Check sheet for the drawn part. Datum: minimum x, y, z corner. Units: mm. A direction names the side the tool comes from. Round coordinates to 2 decimals unless told otherwise and drop trailing zeros. Write each loop counter-clockwise with the first axis right and the second up, starting at its lowest first coordinate (ties: lowest second). Pieces come first, ordered by that corner, then holes. Notation, with made-up numbers: (15.5, 11) - (29.5, 11) arc R16 ccw to (29.5, 39) - close; hole circle Ø3 at (-32.5, 59.25). An arc over 180 degrees is marked (long way). Answer as a JSON object with one key per item and string values. Group by question number.
1) Section check C-C (z = 1.1). Enter the section's corners in (x, y), then the cut area to 3 significant figures.
2) Section check D-D (y = 1.2). Enter the section's corners in (x, z), then the cut area to 3 significant figures.
3) Go/stop test with flat-tipped pins: pin 1 Ø1.5 at (y, z) = (2, 2) entering from +X; pin 2 Ø1 at (x, y) = (4.5, 2) entering from -Z. Record where each tip stops, or that it passes through.
4) Thickness scan on line 1 (Y direction, x = 3, z = 1.8); line 2 (Z direction, x = 3.85, y = 5.5); line 3 (Y direction, x = 1.8, z = 1.6). Record the ranges inside material, lowest first.
5) Set-up check for the marked faces 3 and 4: record each of +Z, -Z, +X, -X, +Y, -Y from which the full face is reachable in a straight line by a thin tool's end or side.
6) Mould release check, pull along Y, two halves, no side actions. Record for the marked faces 1 and 2: +Y half, -Y half, draft (parallel to the pull), parting line (faces both ways), or undercut.
7) Section check A-A (y = 3). Enter the section's corners in (x, z), then the cut area to 3 significant figures.
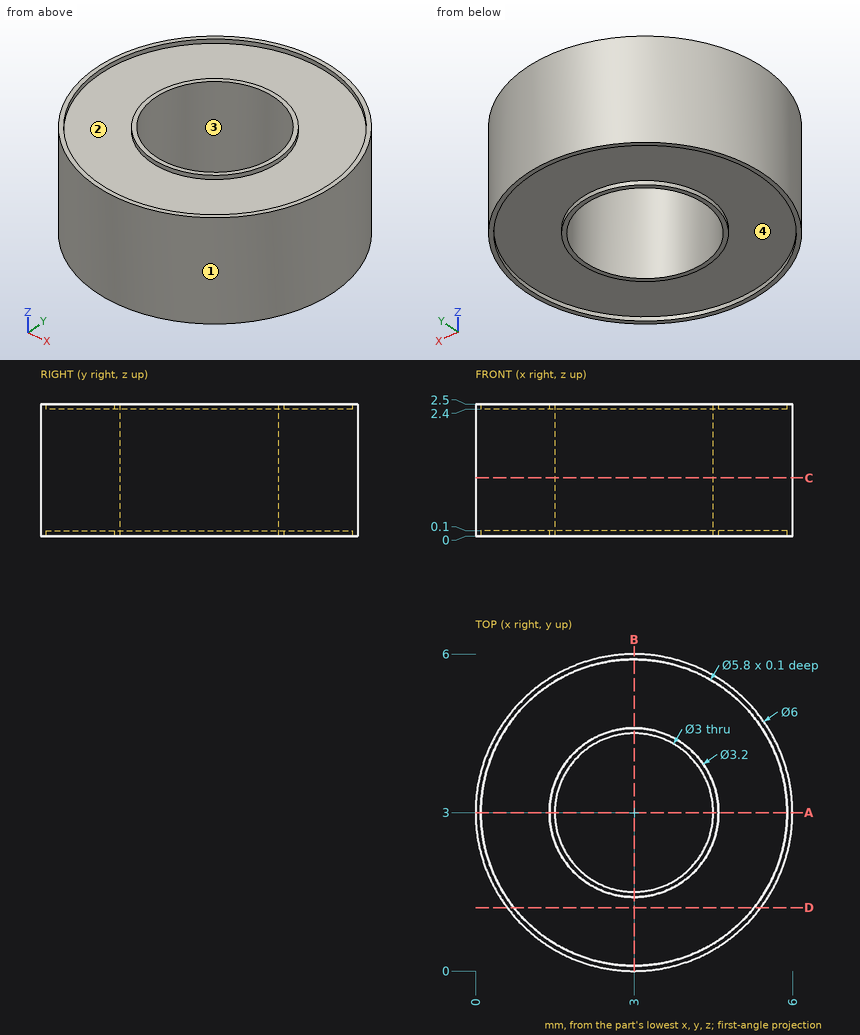
Returned:
{
 "1": {"outline": "circle Ø6 at (3, 3); hole circle Ø3 at (3, 3)", "area": "21.2 mm2"},
 "2": {"outline": "(0.6, 0) - (0.73, 0) - (0.73, 0.1) - (5.27, 0.1) - (5.27, 0) - (5.4, 0) - (5.4, 2.5) - (5.27, 2.5) - (5.27, 2.4) - (0.73, 2.4) - (0.73, 2.5) - (0.6, 2.5) - close", "area": "11.1 mm2"},
 "3": {"pin 1": "x = 5.99", "pin 2": "z = 0"},
 "4": {"line 1": "0 to 1.5, 4.5 to 6", "line 2": "0.1 to 2.4", "line 3": "0.25 to 2.1, 3.9 to 5.75"},
 "5": {"face 3": "+Z, -Z", "face 4": "-Z"},
 "6": {"face 1": "parting line", "face 2": "undercut"},
 "7": {"outline": "(0, 0) - (0.1, 0) - (0.1, 0.1) - (1.4, 0.1) - (1.4, 0) - (1.5, 0) - (1.5, 2.5) - (1.4, 2.5) - (1.4, 2.4) - (0.1, 2.4) - (0.1, 2.5) - (0, 2.5) - close; (4.5, 0) - (4.6, 0) - (4.6, 0.1) - (5.9, 0.1) - (5.9, 0) - (6, 0) - (6, 2.5) - (5.9, 2.5) - (5.9, 2.4) - (4.6, 2.4) - (4.6, 2.5) - (4.5, 2.5) - close", "area": "6.98 mm2"}
}
